```python
from build123d import *

# Parameters (mm, degrees)
CROQUIS1_W              = 730
CROQUIS1_H              = 15
SALIENTE_EXTRUIR1_DEPTH = 40
SALIENTE_EXTRUIR2_DEPTH = 370
CROQUIS3_R              = 2
CORTAR_EXTRUIR1_DEPTH   = 10
CROQUIS4_R              = 2
CORTAR_EXTRUIR2_DEPTH   = 10
CORTAR_EXTRUIR3_START   = -10
CROQUIS5_R              = 2
CORTAR_EXTRUIR3_DEPTH   = 10


with BuildPart() as part:
    # Croquis1 → Saliente-Extruir1 (new body)
    with BuildSketch(Plane.XY):
        Rectangle(CROQUIS1_W, CROQUIS1_H)
    extrude(amount=SALIENTE_EXTRUIR1_DEPTH)

    # Croquis2 → Saliente-Extruir2 (add)
    with BuildSketch(Plane.XY.offset(40)):
        Polygon((-366, -8.5), (-336, -8.5), (-336, -7.5), (-365, -7.5), (-365, 7.5), (-336, 7.5), (-336, 8.5), (-366, 8.5), align=None)
        Polygon((336, 8.5), (366, 8.5), (366, -8.5), (336, -8.5), (336, -7.5), (365, -7.5), (365, 7.5), (336, 7.5), align=None)
    extrude(amount=-SALIENTE_EXTRUIR2_DEPTH)

    # Croquis3 → Cortar-Extruir1 (cut)
    with BuildSketch(Plane(origin=(0, 8.5, 0), x_dir=(1, 0, 0), z_dir=(0, 1, 0))):
        with Locations(Location((351, -20, 0), (0, 0, 270))):
            Circle(CROQUIS3_R)
        with Locations(Location((-351, -20, 0), (0, 0, 270))):
            Circle(CROQUIS3_R)
    extrude(amount=-CORTAR_EXTRUIR1_DEPTH, mode=Mode.SUBTRACT)

    # Croquis4 → Cortar-Extruir2 (cut)
    with BuildSketch(Plane(origin=(366, 0, 0), x_dir=(0, 0, -1), z_dir=(1, 0, 0))):
        with Locations((-30, 0)):
            Circle(CROQUIS4_R)
    extrude(amount=-CORTAR_EXTRUIR2_DEPTH, mode=Mode.SUBTRACT)

    # Croquis5 → Cortar-Extruir3 (cut)
    with BuildSketch(Plane.ZY.offset(366).offset(CORTAR_EXTRUIR3_START)):
        with Locations(Location((30, 0, 0), (0, 0, 180))):
            Circle(CROQUIS5_R)
    extrude(amount=CORTAR_EXTRUIR3_DEPTH, mode=Mode.SUBTRACT)


solid = part.part
```
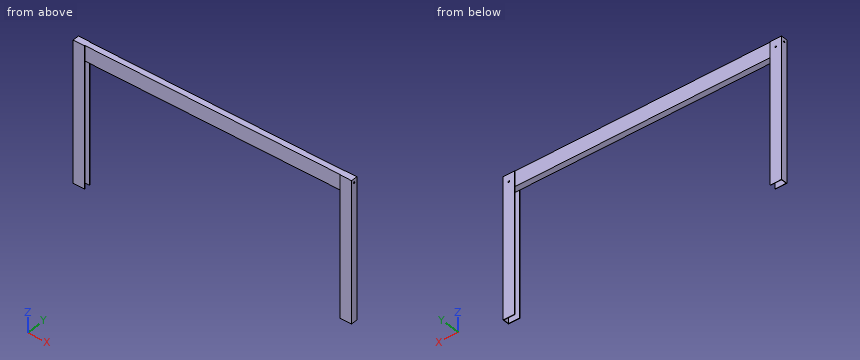
Model file for the job. Use its own axes, mm. Coordinates: 2 decimals unless noted, no trailing zeros. Loops run counter-clockwise (first coordinate to the right, second up) from the corner with the lowest first, then second, coordinate; pieces in that order, holes last. Notation, with made-up numbers: (83.25, 14.25) -> (125.25, 14.25) arc R26 cw to (125.25, 50.25) -> close; hole circle Ø9 at (39, -21.75). An arc over 180 degrees is marked (long way). Answer as a JSON object with one key per item and string values.
Q1. Flat gauge pins, fed straight in: P1, Ø2, axis at x = -214, y = 1, coming from the -Z side; P2, Ø1.2, axis at y = -0.5, z = 31, coming from the +X side; P3, Ø1.2, axis at x = 351, z = 19.5, coming from the +Y side. Where does each tip first touch, or does it go through?
Report:
{"P1": "stops at z = 0", "P2": "stops at x = 356", "P3": "stops at y = -1.5"}
Q2. Probe probe 1 along X at (y, z) = (4.5, 20); probe 2 along Y at (x, z) = (-360, 30); probe 3 along X at (y, z) = (6, -262). List the from-to ranges inside material, lowest first.
Report:
{"probe 1": "x = -366 to -353, -349 to 349, 353 to 366", "probe 2": "y = -8.5 to -2, 2 to 8.5", "probe 3": "x = -366 to -365, 365 to 366"}
Q3. Cut at A-A (z = -303). List the corners of the cut face in (x, y).
Report:
{"outline": "(-366, -8.5) -> (-336, -8.5) -> (-336, -7.5) -> (-365, -7.5) -> (-365, 7.5) -> (-336, 7.5) -> (-336, 8.5) -> (-366, 8.5) -> close; (336, -8.5) -> (366, -8.5) -> (366, 8.5) -> (336, 8.5) -> (336, 7.5) -> (365, 7.5) -> (365, -7.5) -> (336, -7.5) -> close"}
Q4. Cut at B-B (x = -188.5). List the corners of the cut face in (y, z), and give its area (3 significant figures).
Report:
{"outline": "(-7.5, 0) -> (7.5, 0) -> (7.5, 40) -> (-7.5, 40) -> close", "area": "600 mm2"}
